Input: dimensioned drawing with shaded views. Units: mm. Origin: part minimum x, y, z. A direction names the side the tool comes from. Give positions to 0.01 mm unless a question says otherwise; leave off trailing zeros. Loops run counter-clockwise (first coordinate to the right, second up) from the corner with the lowest first, then second, coordinate; pieces in that order, holes last. Notation, with made-up numbers: (-32, -7.5) -> (-9, -7.5) arc R25 cw to (-9, 15.5) -> close; hole circle Ø9 at (37.25, 57). An arc over 180 degrees is marked (long way). Answer in a Markdown table with one row per item. Add a question column.
1) Section query B-B (y = 2.25). Return the cut outline in (x, z) (3 decimals).
2) Section query A-A (x = 2.75). Return the cut outline in (y, z), plus the area to 3 significant figures.
3) Draft query along Y for the marked faces 1, 2 and 3. Return one class per face: +Y half, -Y half, draft (parallel to the pull), parting line (faces both ways), or undercut.
4) Line query: line 1 (X direction, y = 1.75, z = 10.5); line 2 (X direction, y = 8, z = 6.5); line 3 (Y direction, x = 8, z = 11.75). Output: solid intervals per line, ascending. Write a range as from..to.
5) First-contact query: P1, Ø1.6, axis at x = 8, z = 11.5, coming from the +Y side; P2, Ø3, axis at y = 12, z = 7, coming from the -X side; P3, Ø1.5, axis at x = 3, y = 14, coming from the +Z side. Flat tips, straight axial feed; report the tip coordinate or a pass-through.
6) Section query C-C (z = 6.5). Return the cut outline in (x, y), plus the area to 3 significant figures.
7) Access query for the marked faces 4, 5 and 6. Directions: +Z, -Z, +X, -X, +Y, -Y. A direction counts if a zero-diameter tool reaches every point of the face in a straight line with its end or side. Return the directions, or none.
8) Section query D-D (y = 15). Return the cut outline in (x, z).
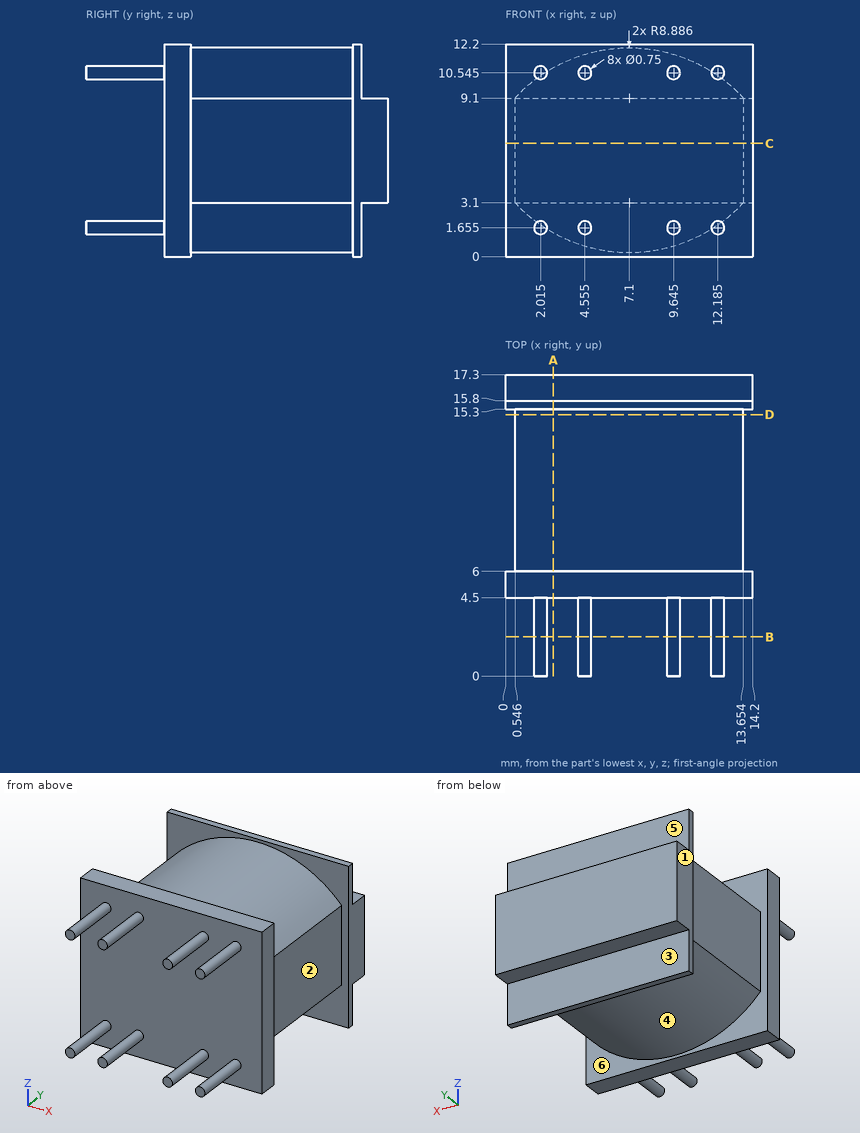
Evaluation:
| question | item | result |
|---|---|---|
| 1 | outline | circle Ø0.75 at (2.015, 1.655); circle Ø0.75 at (2.015, 10.545); circle Ø0.75 at (4.555, 1.655); circle Ø0.75 at (4.555, 10.545); circle Ø0.75 at (9.645, 1.655); circle Ø0.75 at (9.645, 10.545); circle Ø0.75 at (12.185, 1.655); circle Ø0.75 at (12.185, 10.545) |
| 2 | outline | (4.5, 0) -> (6, 0) -> (6, 1.35) -> (15.3, 1.35) -> (15.3, 0) -> (15.8, 0) -> (15.8, 3.1) -> (17.3, 3.1) -> (17.3, 9.1) -> (15.8, 9.1) -> (15.8, 12.2) -> (15.3, 12.2) -> (15.3, 10.85) -> (6, 10.85) -> (6, 12.2) -> (4.5, 12.2) -> close |
| 2 | area | 122 mm² |
| 3 | face 1 | draft |
| 3 | face 2 | undercut |
| 3 | face 3 | +Y half |
| 4 | line 1 | 1.64..2.39, 4.18..4.93, 9.27..10.02, 11.81..12.56 |
| 4 | line 2 | 0.55..13.65 |
| 4 | line 3 | 4.5..15.8 |
| 5 | P1 | y = 15.8 |
| 5 | P2 | x = 0.55 |
| 5 | P3 | z = 11.33 |
| 6 | outline | (0, 4.5) -> (14.2, 4.5) -> (14.2, 6) -> (13.65, 6) -> (13.65, 15.3) -> (14.2, 15.3) -> (14.2, 17.3) -> (0, 17.3) -> (0, 15.3) -> (0.55, 15.3) -> (0.55, 6) -> (0, 6) -> close |
| 6 | area | 172 mm² |
| 7 | face 4 | -Z |
| 7 | face 5 | +Z, +X, -X, +Y |
| 7 | face 6 | none |
| 8 | outline | (0.55, 3.1) arc R8.89 ccw to (13.65, 3.1) -> (13.65, 9.1) arc R8.89 ccw to (0.55, 9.1) -> close |
